Verification items for this drawing (mm, ordinates from the low corner). A direction names the side the tool comes from. Round coordinates to 2 decimals unless told otherwise and drop trailing zeros. Order: outer loops, then holes, each group sorted by start corner. A loop starts at its lowest first (then second) coordinate and runs counter-clockwise, first axis right, second up. Notation, with made-up numbers: (-14, 31) -> (39, 31) arc R21 ccw to (39, 47) -> close; hole circle Ø10 at (48, -1). An arc over 180 degrees is marked (long way). Answer in a Markdown table with one row per item. Add a question column.
1. Sectioned sample at C-C, the plane y = 35.8. Record the boundary of the cut face in (x, z), then the cut area to 3 significant figures.
2. Material ranges on L1, parallel to Y at x = 5.5, z = 6; L2, parallel to Y at x = 23, z = 5.75; L3, parallel to Y at x = 24.05, z = 4, recorded low to high. Write a range as from..to.
3. Access from +Z, -Z, +X, -X, +Y, -Y to the whole of each face (thin tool, end or side, straight path). Record for the marked faces 5, 6 and 7.
4. Sectioned sample at D-D, the plane x = 15.25. Record the boundary of the cut face in (y, z).
5. Sectioned sample at A-A, the plane z = 16. Record the boundary of the cut face in (x, y).
6. Depth check by flat-ended pin: P1, Ø6.5, axis at y = 1.5, z = 5, coming from the -X side; P2, Ø9.5, axis at x = 12.5, z = 6, coming from the +Y side; P3, Ø5.5, axis at x = 12, z = 14, coming from the -Y side. Enter the tip coordinate at first touch or a pass-through.
7. Draft check along Y on the marked faces 1, 2, 3 and 4. Enter one of: +Y half, -Y half, draft (parallel to the pull), parting line (faces both ways), or undercut.
8. Sectioned sample at B-B, the plane x = 18. Record the boundary of the cut face in (y, z).
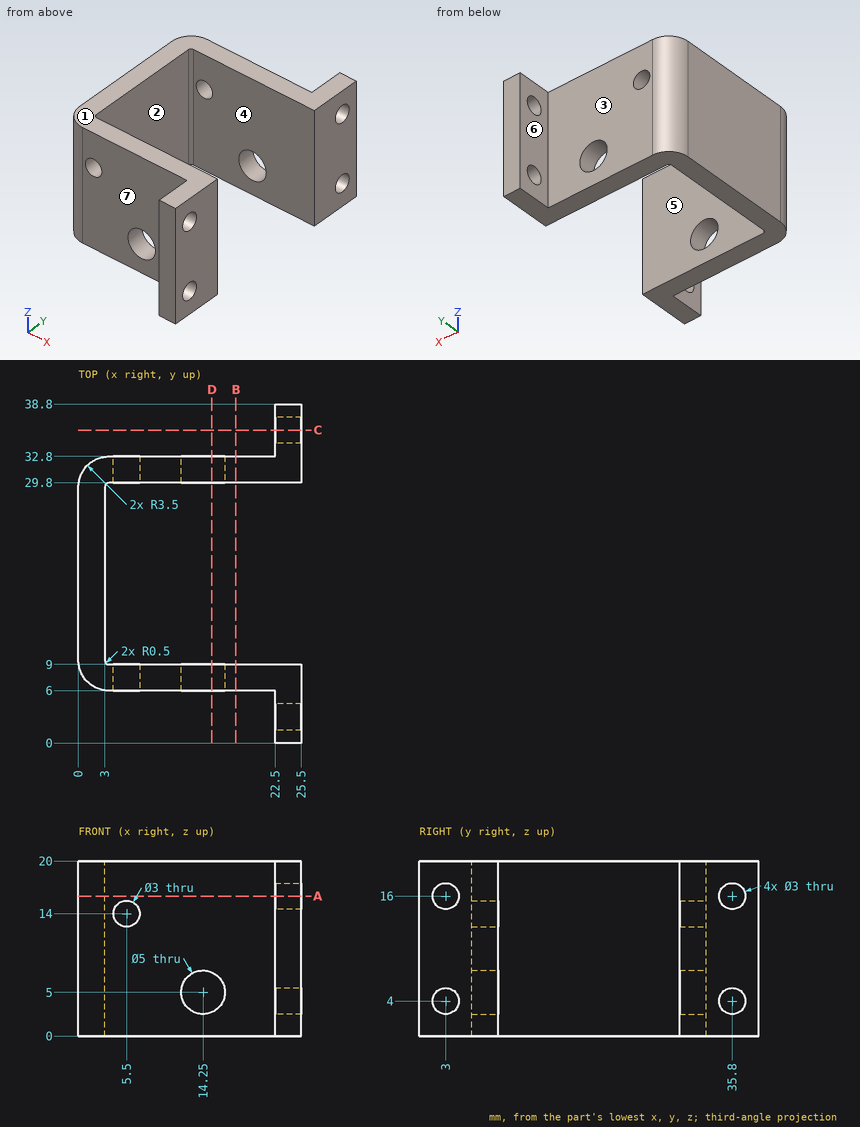
Answer key:
| question | item | result |
|---|---|---|
| 1 | outline | (22.5, 0) -> (25.5, 0) -> (25.5, 2.5) -> (22.5, 2.5) -> close; (22.5, 5.5) -> (25.5, 5.5) -> (25.5, 14.5) -> (22.5, 14.5) -> close; (22.5, 17.5) -> (25.5, 17.5) -> (25.5, 20) -> (22.5, 20) -> close |
| 1 | area | 42.0 mm² |
| 2 | L1 | y = 6..9, 29.8..32.8 |
| 2 | L2 | y = 0..9, 29.8..38.8 |
| 2 | L3 | y = 0..1.5, 4.5..9, 29.8..34.3, 37.3..38.8 |
| 3 | face 5 | +Z, -Z, +X |
| 3 | face 6 | +Z, -Z, -X, +Y |
| 3 | face 7 | +Z, -Z, -X, -Y |
| 4 | outline | (6, 0) -> (9, 0) -> (9, 2.71) -> (6, 2.71) -> close; (6, 7.29) -> (9, 7.29) -> (9, 20) -> (6, 20) -> close; (29.8, 0) -> (32.8, 0) -> (32.8, 2.71) -> (29.8, 2.71) -> close; (29.8, 7.29) -> (32.8, 7.29) -> (32.8, 20) -> (29.8, 20) -> close |
| 5 | outline | (0, 9.5) arc R3.5 ccw to (3.5, 6) -> (22.5, 6) -> (22.5, 4.5) -> (25.5, 4.5) -> (25.5, 9) -> (3.5, 9) arc R0.5 cw to (3, 9.5) -> (3, 29.3) arc R0.5 cw to (3.5, 29.8) -> (25.5, 29.8) -> (25.5, 34.3) -> (22.5, 34.3) -> (22.5, 32.8) -> (3.5, 32.8) arc R3.5 ccw to (0, 29.3) -> close; (22.5, 0) -> (25.5, 0) -> (25.5, 1.5) -> (22.5, 1.5) -> close; (22.5, 37.3) -> (25.5, 37.3) -> (25.5, 38.8) -> (22.5, 38.8) -> close |
| 6 | P1 | stops at x = 22.5 |
| 6 | P2 | stops at y = 32.8 |
| 6 | P3 | stops at y = 6 |
| 7 | face 1 | draft |
| 7 | face 2 | undercut |
| 7 | face 3 | +Y half |
| 7 | face 4 | undercut |
| 8 | outline | (6, 0) -> (9, 0) -> (9, 20) -> (6, 20) -> close; (29.8, 0) -> (32.8, 0) -> (32.8, 20) -> (29.8, 20) -> close |
